The model under review builds one solid part; all positions refer to its coordinate system, in mm. Coordinates: 2 decimals unless noted, no trailing zeros. Order: outer loops, then holes, each group sorted by start corner. A loop starts at its lowest first (then second) coordinate and runs counter-clockwise, first axis right, second up.
```python
from build123d import *

# Parameters (mm, degrees)
CROQUIS1_R              = 200
CROQUIS1_R_2            = 160
CROQUIS1_R_3            = 5.4
SALIENTE_EXTRUIR1_DEPTH = 4
CROQUIS2_R              = 200
CROQUIS2_R_2            = 140
SALIENTE_EXTRUIR2_DEPTH = 4


with BuildPart() as part:
    # Croquis1 → Saliente-Extruir1 (new body)
    with BuildSketch(Plane.XY):
        Circle(CROQUIS1_R)
        Circle(CROQUIS1_R_2, mode=Mode.SUBTRACT)
        with Locations((145.623058987, 105.801345413)):
            Circle(CROQUIS1_R_3, mode=Mode.SUBTRACT)
        with Locations((164.438182376, 73.212595754)):
            Circle(CROQUIS1_R_3, mode=Mode.SUBTRACT)
        with Locations((176.066568132, 37.424104347)):
            Circle(CROQUIS1_R_3, mode=Mode.SUBTRACT)
        with Locations((180, 0)):
            Circle(CROQUIS1_R_3, mode=Mode.SUBTRACT)
        with Locations((176.066568132, -37.424104347)):
            Circle(CROQUIS1_R_3, mode=Mode.SUBTRACT)
        with Locations((164.438182376, -73.212595754)):
            Circle(CROQUIS1_R_3, mode=Mode.SUBTRACT)
        with Locations((145.623058987, -105.801345413)):
            Circle(CROQUIS1_R_3, mode=Mode.SUBTRACT)
        with Locations((120.443509145, -133.766068586)):
            Circle(CROQUIS1_R_3, mode=Mode.SUBTRACT)
        with Locations((90, -155.884572681)):
            Circle(CROQUIS1_R_3, mode=Mode.SUBTRACT)
        with Locations((55.623058987, -171.190172933)):
            Circle(CROQUIS1_R_3, mode=Mode.SUBTRACT)
        with Locations((18.815123388, -179.013941166)):
            Circle(CROQUIS1_R_3, mode=Mode.SUBTRACT)
        with Locations((-18.815123388, -179.013941166)):
            Circle(CROQUIS1_R_3, mode=Mode.SUBTRACT)
        with Locations((-55.623058987, -171.190172933)):
            Circle(CROQUIS1_R_3, mode=Mode.SUBTRACT)
        with Locations((-90, -155.884572681)):
            Circle(CROQUIS1_R_3, mode=Mode.SUBTRACT)
        with Locations((-120.443509145, -133.766068586)):
            Circle(CROQUIS1_R_3, mode=Mode.SUBTRACT)
        with Locations((-145.623058987, -105.801345413)):
            Circle(CROQUIS1_R_3, mode=Mode.SUBTRACT)
        with Locations((-164.438182376, -73.212595754)):
            Circle(CROQUIS1_R_3, mode=Mode.SUBTRACT)
        with Locations((-176.066568132, -37.424104347)):
            Circle(CROQUIS1_R_3, mode=Mode.SUBTRACT)
        with Locations((-180, 0)):
            Circle(CROQUIS1_R_3, mode=Mode.SUBTRACT)
        with Locations((-176.066568132, 37.424104347)):
            Circle(CROQUIS1_R_3, mode=Mode.SUBTRACT)
        with Locations((-164.438182376, 73.212595754)):
            Circle(CROQUIS1_R_3, mode=Mode.SUBTRACT)
        with Locations((-145.623058987, 105.801345413)):
            Circle(CROQUIS1_R_3, mode=Mode.SUBTRACT)
        with Locations((-120.443509145, 133.766068586)):
            Circle(CROQUIS1_R_3, mode=Mode.SUBTRACT)
        with Locations((-90, 155.884572681)):
            Circle(CROQUIS1_R_3, mode=Mode.SUBTRACT)
        with Locations((-55.623058987, 171.190172933)):
            Circle(CROQUIS1_R_3, mode=Mode.SUBTRACT)
        with Locations((-18.815123388, 179.013941166)):
            Circle(CROQUIS1_R_3, mode=Mode.SUBTRACT)
        with Locations((18.815123388, 179.013941166)):
            Circle(CROQUIS1_R_3, mode=Mode.SUBTRACT)
        with Locations((55.623058987, 171.190172933)):
            Circle(CROQUIS1_R_3, mode=Mode.SUBTRACT)
        with Locations((90, 155.884572681)):
            Circle(CROQUIS1_R_3, mode=Mode.SUBTRACT)
        with Locations((120.443509145, 133.766068586)):
            Circle(CROQUIS1_R_3, mode=Mode.SUBTRACT)
    extrude(amount=SALIENTE_EXTRUIR1_DEPTH)

    # Croquis2 → Saliente-Extruir2 (add)
    with BuildSketch(Plane.XY.offset(4)):
        Circle(CROQUIS2_R)
        Circle(CROQUIS2_R_2, mode=Mode.SUBTRACT)
    extrude(amount=SALIENTE_EXTRUIR2_DEPTH)


solid = part.part
```
(1) Wall thickness on probe 1 along X at (y, z) = (166.5, 1.5) (3 decimals); probe 2 along Y at (x, z) = (88.5, 1.5); probe 3 along Z at (x, y) = (30, 143.5): over which ranges is each line inside the solid? List them lowest first.
A:
probe 1: x = -110.805 to -58.299, -52.947 to 52.947, 58.299 to 110.805
probe 2: y = -179.35 to -161.07, -150.7 to -133.3, 133.3 to 150.7, 161.07 to 179.35
probe 3: z = 4 to 8
(2) We need section B-B, the plane y = 0. Write out the cut boundary in (x, z), and give its area (3 significant figures).
A:
outline: (-200, 0) - (-185.4, 0) - (-185.4, 4) - (-174.6, 4) - (-174.6, 0) - (-160, 0) - (-160, 4) - (-140, 4) - (-140, 8) - (-200, 8) - close; (140, 4) - (160, 4) - (160, 0) - (174.6, 0) - (174.6, 4) - (185.4, 4) - (185.4, 0) - (200, 0) - (200, 8) - (140, 8) - close
area: 714 mm2
(3) We need section C-C, the plane x = 90. Write out the cut boundary in (y, z).
A:
outline: (-178.61, 0) - (-161.28, 0) - (-161.28, 4) - (-150.48, 4) - (-150.48, 0) - (-132.29, 0) - (-132.29, 4) - (-107.24, 4) - (-107.24, 8) - (-178.61, 8) - close; (107.24, 4) - (132.29, 4) - (132.29, 0) - (150.48, 0) - (150.48, 4) - (161.28, 4) - (161.28, 0) - (178.61, 0) - (178.61, 8) - (107.24, 8) - close
(4) We need section A-A, the plane x = 0. Write out the cut boundary in (y, z), and give its area (3 significant figures).
A:
outline: (-200, 0) - (-160, 0) - (-160, 4) - (-140, 4) - (-140, 8) - (-200, 8) - close; (140, 4) - (160, 4) - (160, 0) - (200, 0) - (200, 8) - (140, 8) - close
area: 800 mm2
(5) For pin 1 Ø2 at (y, z) = (-69, 5.5) entering from -X; pin 2 Ø3 at (x, y) = (-164.5, -74.5) entering from -Z; pin 3 Ø1.5 at (x, z) = (41.5, 6.5) entering from +Y, all flat-tipped, find the tip position at first contact; note any pin that passes through.
A:
pin 1: stops at x = -188.09
pin 2: stops at z = 4
pin 3: stops at y = 195.8
